Geometry check sheet. Reference: the model listing, model coordinates, mm. A direction names the side the tool comes from. Give positions to 0.01 mm unless a question says otherwise; leave off trailing zeros. Write each loop counter-clockwise with the first axis right and the second up, starting at its lowest first coordinate (ties: lowest second). Pieces come first, ordered by that corner, then holes. Notation, with made-up numbers: (7.5, -14) - (16.5, -14) arc R31 cw to (16.5, 15) - close; hole circle Ø2 at (25, 73.5). An arc over 180 degrees is marked (long way). Write item = value, one per line. Start each with the question number.
(1) Depth check by flat-ended pin: pin 1 Ø0.5 at (y, z) = (8.5, 4) entering from -X; pin 2 Ø3 at (x, y) = (31.5, 6) entering from -Z (3 decimals); pin 3 Ø0.6 at (y, z) = (9.5, 1.5) entering from -X. Enter the tip coordinate at first touch or a pass-through.
(2) Section check C-C, the plane z = -17. Enter the section's corners in (x, y).
(3) Access from +Z, -Z, +X, -X, +Y, -Y to the whole of each face (thin tool, end or side, straight path). Record for faces 1 (the flat face through (111.531, 0, 0)), 2 (the flat face through (9.931, 8, -8)).
(4) Section check B-B, the plane y = -13. Enter the section's corners in (x, z), plus the area to 3 significant figures.
(5) Thickness scan on L1, parallel to X at y = 3, z = 3.5; L2, parallel to Z at x = 22.5, y = 0.5. Record the ranges inside material, lowest first.
(6) Section check A-A, the plane x = 92.5. Enter the section's corners in (y, z) (3 decimals), plus the area to 3 significant figures.
```python
from build123d import *

# Parameters (mm, degrees)
BOSS_EXTRUDE1_DEPTH = 9.4996
CIRPATTERN1_COUNT   = 22


# Read off the part's stored shape, not the designer's step: ThreadSchematic
with BuildPart() as part:
    # ThreadSchematic outline → ThreadSchematic (revolve)
    with BuildSketch(Plane.YX):
        with BuildLine():
            Line((0, 111.5314), (0, 0))
            ThreePointArc((0, 0), (10.887880066, 2.589775097), (19.443700005, 9.804400006))
            Line((19.443700005, 9.804400006), (19.4437, 9.9314))
            Line((19.4437, 9.9314), (11.0998, 9.9314))
            ThreePointArc((11.0998, 9.9314), (9.986248241, 10.392648241), (9.525, 11.5062))
            Line((9.525, 11.5062), (9.525, 111.5314))
            Line((9.525, 111.5314), (0, 111.5314))
        make_face()
    revolve(axis=Axis((0, 0, 0), (1, 0, 0)))

    # Sketch2 → Boss-Extrude1 (add)
    with BuildSketch(Plane(origin=(12.7254, 0, 0), x_dir=(0, 0, -1), z_dir=(1, 0, 0))):
        Polygon((-9.9695, 0), (-9.514107563, -0.455392437), (0, 0), (-9.514107563, 0.455392437), align=None)
    boss_extrude1 = extrude(amount=BOSS_EXTRUDE1_DEPTH)

    # CirPattern1: Boss-Extrude1 ×22 about axis
    cirpattern1_axis = Axis((0, 0, 0), (1, 0, 0))
    for i in range(1, CIRPATTERN1_COUNT):
        add(boss_extrude1.rotate(cirpattern1_axis, i * 360 / CIRPATTERN1_COUNT))


solid = part.part
```
Model answer:
q1.pin_1 = 1.8
q1.pin_2 = -8.395
q1.pin_3 = 1.87
q2.outline = (9.8, -9.44) - (9.93, -9.44) - (9.93, 9.44) - (9.8, 9.44) arc R17.2 ccw to start
q3.face_1 = +Z, -Z, +X, +Y, -Y
q3.face_2 = +X
q4.outline = (9.8, -14.46) - (9.93, -14.46) - (9.93, 14.46) - (9.8, 14.46) arc R20.39 ccw to start
q4.area = 124 mm²
q5.L1 = 0.44 to 111.53
q5.L2 = -9.51 to 9.51
q6.outline = circle Ø19.05 at (0, 0)
q6.area = 285 mm²
